The model under review builds one solid part; all positions refer to its coordinate system, in mm. Face numbers are marked on the shaded views. A direction names the side the tool comes from. Coordinates: 2 decimals unless noted, no trailing zeros. Loops run counter-clockwise (first coordinate to the right, second up) from the corner with the lowest first, then second, coordinate; pieces in that order, holes last. Notation, with made-up numbers: (80.5, 69) - (114.5, 69) arc R26 ccw to (114.5, 90) - close; hole circle Ø7 at (44.25, -6.75). An arc over 180 degrees is marked (long way). Use a Markdown table: item, result. Add a question column.
1) To check wall thickness, follow L1, parallel to Z at x = -13, y = 7; L2, parallel to Y at x = -16.5, z = -35; L3, parallel to Z at x = 38, y = -17. State the ranges of each line that lie inside material, in increasing order. Write a range as [from, to].
2) Add section B-B, the plane x = -15. Give the boundary of the cut face in (y, z).
3) Add section A-A, the plane y = 2.5. Give the boundary of the cut face in (x, z).
4) Clearance check with flat-ended pins moving along their axes: pin 1 (1.1 mm diameter, centred on y = 24.5, z = 1.5, fed in from -X); pin 2 (17 mm diameter, centred on y = -10.5, z = -11, fed in from -X); pin 3 (3 mm diameter, centred on x = -22.5, z = -29.5, fed in from +Y); pin 4 (8.5 mm diameter, centred on x = 3, y = 6.5, fed in from +Z). State where each tip first meets the part, or that it passes through.
5) Add section D-D, the plane y = -8. Give the boundary of the cut face in (x, z).
6) The part is to be moulded in two halves that separate along Y. For the marked faces 1, 2, 3 and 4, say which applies: pulls with the +Y half, pulls with the -Y half, needs draft (parallel to the pull), parting line crosses it, or undercut.
7) For the marked faces 5, 6, 7, 8 and 9, list the 3-axis set-ups (+Z, -Z, +X, -X, +Y, -Y) from which the entire face can be reached by the end or side of a thin tool; tool diameter is ignored.
8) Add section C-C, the plane z = 32.5. Give the boundary of the cut face in (x, y), and give its area (3 significant figures).
```python
from build123d import *

# Parameters (mm, degrees)
F0_W      = 82.406614
F0_H      = 96.04887
F1_DEPTH  = 25.4
F2_W      = 73.741935
F2_H      = 15.301453
F3_DEPTH  = 92.202
F4_W      = 41.848549
F4_H      = 3.502742
F5_DEPTH  = 33.782
F7_DEPTH  = 58.928
F9_DEPTH  = 50.292
F10_W     = 14.748386
F10_H     = 6.452419
F11_DEPTH = 25.4
F12_W     = 1.843547
F12_H     = 87.199841
F13_DEPTH = 3.048
F14_R     = 9.422481
F15_DEPTH = 88.9
F16_R     = 9.422481
F17_DEPTH = 1.524


with BuildPart() as f1:
    # F0 (on Front) → F1 (new body)
    with BuildSketch(Plane.XZ):
        with Locations((1.474841, -4.240159)):
            Rectangle(F0_W, F0_H)
    extrude(amount=F1_DEPTH)

    # F2 (on face) → F3 (cut)
    with BuildSketch(Plane.XY.offset(43.784276)):
        with Locations((1.751371, -12.351774)):
            Rectangle(F2_W, F2_H)
    extrude(amount=-F3_DEPTH, mode=Mode.SUBTRACT)

    # F4 (on face) → F5 (join)
    with BuildSketch(Plane(origin=(0, 0, 0), x_dir=(-1, 0, 0), z_dir=(0, 1, 0))):
        with Locations((0.184355, 1.751371)):
            Rectangle(F4_W, F4_H)
        with Locations((0.184355, -15.670161)):
            Rectangle(F4_W, F4_H)
    extrude(amount=F5_DEPTH)

    # F6 (on face) → F7 (cut)
    with BuildSketch(Plane.YZ.offset(20.73992)):
        Polygon((33.782, 3.502742), (16.891, 3.502742), (33.782, 0), align=None)
    extrude(amount=-F7_DEPTH, mode=Mode.SUBTRACT)

    # F8 (on face) → F9 (cut)
    with BuildSketch(Plane.YZ.offset(20.73992)):
        Polygon((33.782, -13.91879), (16.891, -17.421532), (33.782, -17.421532), align=None)
    extrude(amount=-F9_DEPTH, mode=Mode.SUBTRACT)

    # F10 (on face) → F11 (cut)
    with BuildSketch(Plane(origin=(0, 0, -52.264594), x_dir=(1, 0, 0), z_dir=(0, 0, -1))):
        with Locations((1.75137, 13.457904)):
            Rectangle(F10_W, F10_H)
    extrude(amount=-F11_DEPTH, mode=Mode.SUBTRACT)

    # F12 (on face) → F13 (join)
    with BuildSketch(Plane(origin=(-39.728466, 0, 0), x_dir=(0, -1, 0), z_dir=(-1, 0, 0))):
        with Locations((11.679495, -6.745199)):
            Rectangle(F12_W, F12_H)
    extrude(amount=F13_DEPTH)

    # F14 (on face) → F15 (join)
    with BuildSketch(Plane.XY.offset(36.854722)):
        with BuildLine():
            Line((-42.776466, -12.601268), (-42.776466, -10.757721))
            ThreePointArc((-42.776466, -10.757721), (-65.724916, -11.679494), (-42.776466, -12.601268))
        make_face()
        with Locations((-54.267689, -11.679494)):
            Circle(F14_R, mode=Mode.SUBTRACT)
    extrude(amount=-F15_DEPTH)

    # F16 (on face) → F17 (join)
    with BuildSketch(Plane(origin=(0, 0, -52.045278), x_dir=(1, 0, 0), z_dir=(0, 0, -1))):
        with Locations((-54.267689, 11.679494)):
            Circle(F16_R)
    extrude(amount=-F17_DEPTH)


solid = f1.part
```
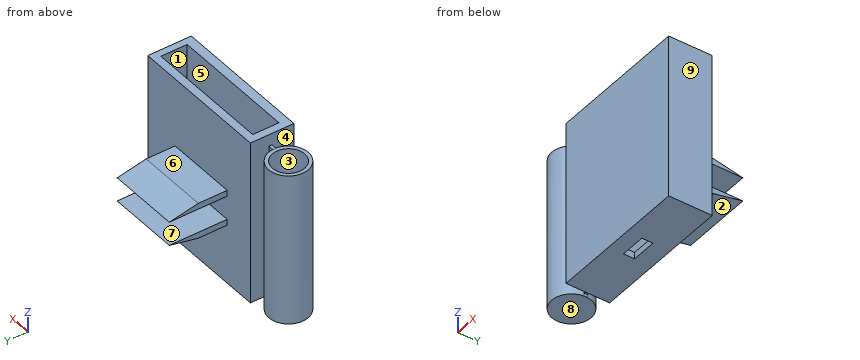
From the geometry:
| question | item | result |
|---|---|---|
| 1 | L1 | z = [-17.42, -13.92], [0, 3.5] |
| 1 | L2 | y = [-25.4, -20], [-4.7, 0] |
| 1 | L3 | z = [-52.26, -48.42] |
| 2 | outline | (-25.4, -52.26) - (0, -52.26) - (0, -17.42) - (16.89, -17.42) - (33.78, -13.92) - (0, -13.92) - (0, 0) - (33.78, 0) - (16.89, 3.5) - (0, 3.5) - (0, 43.78) - (-4.7, 43.78) - (-4.7, -48.42) - (-20, -48.42) - (-20, 43.78) - (-25.4, 43.78) - close |
| 3 | outline | (-21.11, -17.42) - (20.74, -17.42) - (20.74, -13.92) - (-21.11, -13.92) - close; (-21.11, 0) - (20.74, 0) - (20.74, 3.5) - (-21.11, 3.5) - close |
| 4 | pin 1 | stops at x = -21.11 |
| 4 | pin 2 | stops at x = -65.72 |
| 4 | pin 3 | stops at y = 0 |
| 4 | pin 4 | stops at z = 3.5 |
| 5 | outline | (-65.12, -52.05) - (-43.34, -52.05) - (-43.34, 36.85) - (-45.59, 36.85) - (-45.59, -50.52) - (-62.94, -50.52) - (-62.94, 36.85) - (-65.12, 36.85) - close; (-39.73, -52.26) - (42.68, -52.26) - (42.68, 43.78) - (38.62, 43.78) - (38.62, -48.42) - (-35.12, -48.42) - (-35.12, 43.78) - (-39.73, 43.78) - close |
| 6 | face 1 | undercut |
| 6 | face 2 | pulls with the +Y half |
| 6 | face 3 | undercut |
| 6 | face 4 | needs draft |
| 7 | face 5 | +Z |
| 7 | face 6 | +Z, +X, -X, +Y |
| 7 | face 7 | +X, -X, +Y |
| 7 | face 8 | -Z, -X, +Y, -Y |
| 7 | face 9 | +Z, -Z, +X, +Y, -Y |
| 8 | outline | (-42.78, -12.6) - (-39.73, -12.6) - (-39.73, -25.4) - (42.68, -25.4) - (42.68, 0) - (-39.73, 0) - (-39.73, -10.76) - (-42.78, -10.76) arc R11.49 ccw (long way) to start; hole circle Ø18.84 at (-54.27, -11.68); hole (-35.12, -20) - (38.62, -20) - (38.62, -4.7) - (-35.12, -4.7) - close |
| 8 | area | 1,110 mm^2 |
